The model under review builds one solid part; all positions refer to its coordinate system, in mm. A direction names the side the tool comes from. Coordinates: 2 decimals unless noted, no trailing zeros. Loops run counter-clockwise (first coordinate to the right, second up) from the corner with the lowest first, then second, coordinate; pieces in that order, holes last. Notation, with made-up numbers: M 29.25,-7.75 L 59.25,-7.75 A9 cw 59.25,-0.75 Z; hole C 36,14.5 d3. An arc over 180 degrees is marked long. Use CSV: the item, a comma, the result in double quotes. Start each with the question number.
from build123d import *

# Parameters (mm, degrees)
F0_R     = 11.075
F2_DEPTH = 8.5
F3_COUNT = 4


# Not quite as in the source:
# - a feature names something its author has since deleted; it is built from what else it names


with BuildPart() as f2:
    # F0 (on Top) → F2 (new body)
    with BuildSketch(Plane.XY):
        with BuildLine():
            Line((-7.6826518036, 18.0394667333), (-8.7891866596, 12.1552539201))
            ThreePointArc((-8.7891866596, 12.1552539201), (0, -15), (8.7891866596, 12.1552539201))
            Line((8.7891866596, 12.1552539201), (7.6826518036, 18.0394667333))
            ThreePointArc((7.6826518036, 18.0394667333), (7.6938199579, 18.4608846247), (7.8776597121, 18.840253458))
            ThreePointArc((7.8776597121, 18.840253458), (8.9888115293, 29.3819250667), (0, 35))
            Line((0, 35), (-25, 35))
            ThreePointArc((-25, 35), (-25.2828427125, 34.8828427125), (-25.4, 34.6))
            Line((-25.4, 34.6), (-25.4, 34.1))
            ThreePointArc((-25.4, 34.1), (-25.2534392204, 33.7905350399), (-24.9211571922, 33.7078472088))
            ThreePointArc((-24.9211571922, 33.7078472088), (-15.6786460864, 32.0797048321), (-9.9925313497, 24.6135841297))
            ThreePointArc((-9.9925313497, 24.6135841297), (-9.3898226238, 21.5603443352), (-7.8776597121, 18.840253458))
            ThreePointArc((-7.8776597121, 18.840253458), (-7.6938199579, 18.4608846247), (-7.6826518036, 18.0394667333))
        make_face()
        Circle(F0_R, mode=Mode.SUBTRACT)
        Polygon((0, 33.2561088494), (7.15, 29.1280544247), (7.15, 20.8719455753), (0, 16.7438911506), (-7.15, 20.8719455753), (-7.15, 29.1280544247), align=None, mode=Mode.SUBTRACT)
    extrude(amount=F2_DEPTH)

    # F3: F2 ×4 about axis
    f3_axis = Axis((0, 0, 16.6777409613), (0, 0, 1))


with BuildPart() as f2_1:
    add(f2.part)
    for i in range(1, F3_COUNT):
        add(f2.part.rotate(f3_axis, i * 360 / F3_COUNT))


solid = f2_1.part
1. Add section C-C (y = 23). Write out the cut boundary in (x, z).
2. Insertion check: pin 1 Ø4 at (x, z) = (-25.5, 5.5) entering from -Y; pin 2 Ø5 at (y, z) = (-22.5, 6.5) entering from +X; pin 3 Ø3 at (y, z) = (-28, 3.5) entering from -X. Each pin has a flat end and moves straight along its axis. Give the tip position at first contact, or say it passes through.
3. Add section B-B (x = -2). Write out the cut boundary in (y, z), plus the area to 3 significant figures.
4. Add section D-D (x = 26.5). Write out the cut boundary in (y, z), plus the area to 3 significant figures.
5. To check wall thickness, follow line 1 along Y through (x, z) = (0, 2.25) (3 decimals); line 2 along X through (y, z) = (-6, 3.5); line 3 along Y through (x, z) = (17, 3). State the ranges of each line that lie inside material, in increasing order.
6. Add section A-A (y = -14.5). Write out the cut boundary in (x, z), plus the area to 3 significant figures.
7. Draft analysis for pull direction X (two halves, no side actions). For faces 6 (the flat face through (8.228, -15.139, 4.19)), 7 (the flat face through (-7.15, -25, 4)), 8 (the flat face through (12, -35, 4)), state which applies: released by +X, released by -X, zero draft, split by the parting line, or undercut.
8. For faces 1 (the cylindrical face through (9.405, -21.601, 4.19)), 2 (the flat face through (-3.63, -18.84, 4.19)), 3 (the flat face through (15.139, 8.228, 4.19)), 4 (the flat face through (-8.228, 15.139, 4.19)), 5 (the flat face through (-10.2, 5.3, 8.5)), list the 3-axis set-ups (+Z, -Z, +X, -X, +Y, -Y) from which the entire face can be reached by the end or side of a thin tool; tool diameter is ignored.
Solved:
1,outline,"M -9.8,0 L -7.15,0 L -7.15,8.5 L -9.8,8.5 Z; M 7.15,0 L 9.8,0 L 9.8,8.5 L 7.15,8.5 Z; M 33.95,0 L 35,0 L 35,8.5 L 33.95,8.5 Z"
2,pin 1,"stops at y = -11.21"
2,pin 2,"stops at x = 10.11"
2,pin 3,"stops at x = -9.89"
3,outline,"M -34.8,0 L -32.1,0 L -32.1,8.5 L -34.8,8.5 Z; M -17.9,0 L -10.89,0 L -10.89,8.5 L -17.9,8.5 Z; M 10.89,0 L 17.9,0 L 17.9,8.5 L 10.89,8.5 Z; M 32.1,0 L 35,0 L 35,8.5 L 32.1,8.5 Z"
3,area,"167 mm^2"
4,outline,"M -9.89,0 L -7.15,0 L -7.15,8.5 L -9.89,8.5 Z; M 7.15,0 L 10.69,0 L 10.69,8.5 L 7.15,8.5 Z"
4,area,"53.4 mm^2"
5,line 1,"y = -35 to -33.256, -16.744 to -11.075, 11.075 to 16.744, 33.256 to 35"
5,line 2,"x = -35 to -29.79, -20.21 to -9.31, 9.31 to 20.21, 29.79 to 33"
5,line 3,"y = -35 to -32.78, -7.88 to -0.44, 0.44 to 7.88"
6,outline,"M -35,0 L -31.27,0 L -31.27,8.5 L -35,8.5 Z; M -8.35,0 L 8.35,0 L 8.35,8.5 L -8.35,8.5 Z"
6,area,"174 mm^2"
7,face 6,"released by +X"
7,face 7,"undercut"
7,face 8,"zero draft"
8,face 1,"+Z, -Z, +X"
8,face 2,"+Z, -Z"
8,face 3,"+Z, -Z, +Y"
8,face 4,"+Z, -Z, -X"
8,face 5,"+Z, +X, -X, +Y, -Y"
